Input: part model. Units: mm. Frame: model coordinates. A direction names the side the tool comes from. Give positions to 0.01 mm unless a question says otherwise; leave off trailing zeros. Loops run counter-clockwise (first coordinate to the right, second up) from the corner with the lowest first, then second, coordinate; pieces in that order, holes last. Notation, with made-up numbers: (30.25, -30) - (81.25, -30) arc R23 cw to (81.25, -1) - close; hole circle Ø2 at (8.5, 78). An arc over 180 degrees is marked (long way). Answer as a JSON object with one key per item and string values.
from build123d import *

# Parameters (mm, degrees)
BOSS_EXTRUDE1_DEPTH = 12.7
SKETCH2_R           = 38.1
CUT_EXTRUDE1_DEPTH  = 2.54


with BuildPart() as part:
    # Sketch1 → Boss-Extrude1 (new body)
    with BuildSketch(Plane(origin=(0, 0, 0), x_dir=(1, 0, 0), z_dir=(0, 1, 0))):
        Polygon((-609.6, 304.8), (-304.8, 609.6), (304.8, 609.6), (609.6, 304.8), (609.6, -304.8), (304.8, -609.6), (-304.8, -609.6), (-609.6, -304.8), align=None)
    extrude(amount=BOSS_EXTRUDE1_DEPTH)

    # Sketch2 → Cut-Extrude1 (cut)
    with BuildSketch(Plane(origin=(0, 12.7, 0), x_dir=(1, 0, 0), z_dir=(0, 1, 0))):
        Circle(SKETCH2_R)
    extrude(amount=-CUT_EXTRUDE1_DEPTH, mode=Mode.SUBTRACT)


solid = part.part
Item 1: Access query for faces 1 (the face through (-1, 10.16, -1)), 2 (the face through (-455.1, 6.3, 459.3)). Directions: +Z, -Z, +X, -X, +Y, -Y. A direction counts if a zero-diameter tool reaches every point of the face in a straight line with its end or side. Return the directions, or none.
Geometry check:
{"face 1": "+Y", "face 2": "+Z, -X, +Y, -Y"}
Item 2: Cut plane B-B (x = -479.5). Return loops of the section in (y, z), then the cut area to 3 significant figures.
Geometry check:
{"outline": "(0, -434.9) - (12.7, -434.9) - (12.7, 434.9) - (0, 434.9) - close", "area": "11,000 mm2"}
Item 3: Material intervals for line 1 (X direction, y = 11.25, z = 0); line 2 (Z direction, x = 545, y = 3.25), sorted ascending. Write a range as [from, to].
Geometry check:
{"line 1": "x = [-609.6, -38.1], [38.1, 609.6]", "line 2": "z = [-369.4, 369.4]"}
Item 4: Cut plane C-C (z = 499). Return loops of the section in (x, y), then the cut area to 3 significant figures.
Geometry check:
{"outline": "(-415.4, 0) - (415.4, 0) - (415.4, 12.7) - (-415.4, 12.7) - close", "area": "10,600 mm2"}
Item 5: Contact query for a flat-ended pin moving along its axis: P1, Ø4, axis at x = 372.5, z = 251.5, coming from the -Y side. Output: stop coordinate, or through.
Geometry check:
{"P1": "stops at y = 0"}
Item 6: Cut plane A-A (y = 7.75). Return loops of the section in (x, z), then the cut area to 3 significant figures.
Geometry check:
{"outline": "(-609.6, -304.8) - (-304.8, -609.6) - (304.8, -609.6) - (609.6, -304.8) - (609.6, 304.8) - (304.8, 609.6) - (-304.8, 609.6) - (-609.6, 304.8) - close", "area": "1,300,000 mm2"}
Item 7: Mould query, pull axis Z, two halves, no side actions, for faces 3 (the face through (-30.235, 11.448, 23.183)), 4 (the face through (9, 0, -9)), 5 (the face through (-459.3, 6.3, -455.1)), 6 (the face through (459.3, 6.3, 455.1)). Classes: released by +Z, released by -Z, zero draft, split by the parting line, or undercut.
Geometry check:
{"face 3": "undercut", "face 4": "zero draft", "face 5": "released by -Z", "face 6": "released by +Z"}
